Could you check a few things on this model? Use its own coordinates, in mm. Coordinates: 2 decimals unless noted, no trailing zeros. Loops run counter-clockwise (first coordinate to the right, second up) from the corner with the lowest first, then second, coordinate; pieces in that order, holes last. Notation, with made-up numbers: (25.25, -14) - (68.25, -14) arc R29 ccw to (68.25, 21) - close; hole circle Ø8 at (-2.75, 71). An arc over 180 degrees is marked (long way). One line per item, written item: value. Start each with the question number.
(1) If we section it at C-C on z = -2.5: Write out the boundary of the cut face in (x, y) (3 decimals), then the cut area to 3 significant figures.
(2) I'm going to push flat-ended pins straight in: P1, Ø1.5, axis at y = -5, z = -0.5, coming from the +X side; P2, Ø3, axis at y = -13, z = 1, coming from the -X side; P3, Ø5.5, axis at x = 0, y = 0, coming from the -Z side; P4, Ø4, axis at x = 4.5, z = -3, coming from the +Y side. Where does each tip first touch, or does it pass through?
(3) If we mould it in two halves opening along X, with no side actions, what happens to faces 1 (the face through (0, 4, 4.762)), 2 (the face through (18.597, 4.13, 3.155)), 3 (the face through (-1.93, -2.52, -0.07))? For each: pulls with the +X half, pulls with the -X half, needs draft (parallel to the pull), parting line crosses it, or undercut.
(4) If I drill on line 1 along X through (y, z) = (0, 2.5) (3 decimals); line 2 along X through (y, z) = (0, 0.75) (3 decimals); line 3 along Z through (x, y) = (17.5, -3.5), over which ranges is the centre line in solid material (lowest first)? Write a range as from..to.
```python
from build123d import *

# Parameters (mm, degrees)
SKETCH2_R          = 3.175
CUT_EXTRUDE1_DEPTH = 9.525


with BuildPart() as part:
    # Sketch1 → Revolve1 (revolve)
    with BuildSketch(Plane(origin=(0, 0, 0), x_dir=(0, 0, -1), z_dir=(1, 0, 0)), mode=Mode.PRIVATE) as revolve1_sk:
        with BuildLine():
            Line((1.592452886, 19.05), (4.7625, 19.05))
            Line((4.7625, 19.05), (4.7625, 0))
            Line((4.7625, 0), (-4.7625, 0))
            Line((-4.7625, 0), (-4.7625, 19.05))
            Line((-4.7625, 19.05), (-1.592452886, 19.05))
            Line((-1.592452886, 19.05), (-1.581459083, 18.924340258))
            ThreePointArc((-1.581459083, 18.924340258), (0, 17.4752), (1.581459083, 18.924340258))
            Line((1.581459083, 18.924340258), (1.592452886, 19.05))
        make_face()
    revolve(revolve1_sk.sketch.rotate(Axis((0, 0, 4.7625), (0, 0, -1)), 180), axis=Axis((0, 0, 4.7625), (0, 0, -1)))

    # Sketch2 → Cut-Extrude1 (cut)
    with BuildSketch(Plane(origin=(0, 0, -4.7625), x_dir=(-1, 0, 0), z_dir=(0, 0, -1))):
        with Locations(Location((0, 0, 0), (0, 0, 90))):
            Circle(SKETCH2_R)
    extrude(amount=-CUT_EXTRUDE1_DEPTH, mode=Mode.SUBTRACT)


solid = part.part
```
Values:
1. outline: circle Ø38.1 at (0, 0); hole circle Ø6.35 at (0, 0)
1. area: 1,110 mm2
2. P1: stops at x = 17.4
2. P2: stops at x = -15.09
2. P3: passes through
2. P4: stops at y = 18.89
3. face 1: needs draft
3. face 2: parting line crosses it
3. face 3: undercut
4. line 1: x = -19.05..-3.175, 3.175..19.05
4. line 2: x = -17.664..-3.175, 3.175..17.664
4. line 3: z = -4.76..-1.02, 1.02..4.76
